from build123d import *

# Parameters (mm, degrees)
SKETCH2_R           = 18.5
SKETCH2_R_2         = 2
BOSS_EXTRUDE1_DEPTH = 2
SKETCH5_W           = 68.697937928
SKETCH5_H           = 35.271008104
CUT_EXTRUDE1_DEPTH  = 31


with BuildPart() as part:
    # Sketch2 → Boss-Extrude1 (new body)
    with BuildSketch(Plane(origin=(0, 0, 0), x_dir=(1, 0, 0), z_dir=(0, 1, 0))):
        with BuildLine():
            ThreePointArc((30, 2), (29.414213562, 3.414213562), (28, 4))
            Line((28, 4), (21.633307653, 4))
            ThreePointArc((21.633307653, 4), (0, 22), (-21.633307653, 4))
            Line((-21.633307653, 4), (-28, 4))
            ThreePointArc((-28, 4), (-29.414213562, 3.414213562), (-30, 2))
            Line((-30, 2), (-30, -2))
            ThreePointArc((-30, -2), (-29.414213562, -3.414213562), (-28, -4))
            Line((-28, -4), (-21.633307653, -4))
            ThreePointArc((-21.633307653, -4), (0, -22), (21.633307653, -4))
            Line((21.633307653, -4), (28, -4))
            ThreePointArc((28, -4), (29.414213562, -3.414213562), (30, -2))
            Line((30, -2), (30, 2))
        make_face()
        Circle(SKETCH2_R, mode=Mode.SUBTRACT)
        with Locations((27, 0)):
            Circle(SKETCH2_R_2, mode=Mode.SUBTRACT)
        with Locations((-27, 0)):
            Circle(SKETCH2_R_2, mode=Mode.SUBTRACT)
    extrude(amount=BOSS_EXTRUDE1_DEPTH)

    # Sketch4 → Revolve1 (revolve)
    with BuildSketch(Plane.XY):
        with BuildLine():
            Line((-21.633307653, 0), (-18.5, 0))
            ThreePointArc((-18.5, 0), (-17.823557637, 4.956893497), (-15.843698038, 9.551294806))
            Line((-15.843698038, 9.551294806), (-17.782437649, 12.320101917))
            ThreePointArc((-17.782437649, 12.320101917), (-20.648159052, 6.453954428), (-21.633307653, 0))
        make_face()
    revolve(axis=Axis((0, 21.633307653, 0), (0, -1, 0)))

    # Sketch5 → Cut-Extrude1 (cut, through all)
    with BuildSketch(Plane(origin=(0, 0, 0), x_dir=(0, 0, -1), z_dir=(1, 0, 0))):
        Rectangle(SKETCH5_W, SKETCH5_H)
    extrude(amount=-CUT_EXTRUDE1_DEPTH, mode=Mode.SUBTRACT)


solid = part.part
Source: CAD feature listing. Evaluate the final solid. Frame: model axes, mm. A direction names the side the tool comes from. Round coordinates to 2 decimals unless told otherwise and drop trailing zeros. Loops run counter-clockwise (first coordinate to the right, second up) from the corner with the lowest first, then second, coordinate; pieces in that order, holes last. Notation, with made-up numbers: (-38, 30) -> (3, 30) arc R13 cw to (3, 34) -> close; hole circle Ø4 at (70.5, 35). An arc over 180 degrees is marked (long way). Answer as a JSON object with one key per item and string values. Group by question number.
Q1. Section query D-D (y = 5.75). Output: boundary loops of the cut face in (x, z).
Q2. Contact query for flat-ended pins moving along their axis: P1, Ø3, axis at y = 5, z = -2, coming from the -X side; P2, Ø1, axis at x = 26, y = 1, coming from the +Z side; P3, Ø1, axis at y = 10.5, z = -3.5, coming from the +X side. Output: stop coordinate, or through.
Q3. Ray query, line 1 (Z direction, x = 27, y = 0.5); line 2 (Z direction, x = 1.75, y = 9.25); line 3 (X direction, y = 0.6, z = 0). Return the intervals inside material, ascending. Write a range as from..to.
Q4. Section query A-A (x = 27). Output: boundary loops of the cut face in (y, z).
Q5. Access query for faces 1 (the flat face through (25, 1, -4)), 2 (the flat face through (0, 6, -19)), 3 (the flat face through (22, 2, 0)). Directions: +Z, -Z, +X, -X, +Y, -Y. A direction counts if a zero-diameter tool reaches every point of the face in a straight line with its end or side. Return the directions, or none.
Q6. Section query C-C (x = 24). Output: boundary loops of the cut face in (y, z), plus the area to 3 significant figures.
Q7. Mould query, pull axis Z, two halves, no side actions, for faces 4 (the flat face through (25, 1, 4)), 5 (the flat face through (19, 0, 0)), 6 (the cylindrical face through (28.908, 0.986, -0.601)), 7 (the conical face through (15.96, 9.72, -0.35)). Classes: pulls with the +Z half, pulls with the -Z half, needs draft (parallel to the pull), parting line crosses it, or undercut.
Q8. Section query B-B (z = 0). Output: boundary loops of the cut face in (x, y).
Completed:
{
 "1": {"outline": "(0, -20.86) arc R20.86 ccw to (0, 20.86) -> (0, 17.58) arc R17.58 cw to (0, -17.58) -> close"},
 "2": {"P1": "x = 17.17", "P2": "z = 4", "P3": "x = 18.88"},
 "3": {"line 1": "-4..-2, 2..4", "line 2": "-19.48..-15.93, 15.93..19.48", "line 3": "18.49..25, 29..30"},
 "4": {"outline": "(0, -4) -> (2, -4) -> (2, -2) -> (0, -2) -> close; (0, 2) -> (2, 2) -> (2, 4) -> (0, 4) -> close"},
 "5": {"face 1": "-Z, +X, +Y, -Y", "face 2": "+Z, -Z, -X, +Y, -Y", "face 3": "+X, +Y"},
 "6": {"outline": "(0, -4) -> (2, -4) -> (2, 4) -> (0, 4) -> close", "area": "16.0 mm²"},
 "7": {"face 4": "pulls with the +Z half", "face 5": "needs draft", "face 6": "undercut", "face 7": "undercut"},
 "8": {"outline": "(15.84, 9.55) arc R18.5 cw to (18.5, 0) -> (25, 0) -> (25, 2) -> (21.54, 2) arc R21.63 ccw to (17.78, 12.32) -> close; (29, 0) -> (30, 0) -> (30, 2) -> (29, 2) -> close"}
}
